Model file for the job. Use its own axes, mm. A direction names the side the tool comes from. Round coordinates to 2 decimals unless told otherwise and drop trailing zeros. Loops run counter-clockwise (first coordinate to the right, second up) from the corner with the lowest first, then second, coordinate; pieces in that order, holes last. Notation, with made-up numbers: M 22,71 L 58,71 A23 ccw 58,81 Z; hole C 88,49.25 d10. An arc over 180 degrees is marked long. Answer in a Markdown table with one row per item.
Autodesk Inventor part; units mm, degrees
ref_plane "YZ Plane" through (0, 0, 0) normal (1, 0, 0) x (0, 1, 0)
ref_plane "XZ Plane" through (0, 0, 0) normal (0, 1, 0) x (-1, 0, 0)
ref_plane "XY Plane" through (0, 0, 0) normal (0, 0, 1) x (1, 0, 0)
sketch "Эскиз1" plane through (0, 0, 0) normal (0, 1, 0) x (-1, 0, 0)
  line L0 (15, -5) -> (-15, -5)
  line L1 (-15, -5) -> (-15, 5)
  line L2 (-15, 5) -> (15, 5)
  line L3 (15, 5) -> (15, -5)
  line L4 (-15, -5) -> (15, 5) construction
  line L5 (15, -5) -> (-15, 5) construction
  line L6 (-13, -3) -> (13, -3)
  line L7 (13, -3) -> (13, 3)
  line L8 (13, 3) -> (-13, 3)
  line L9 (-13, 3) -> (-13, -3)
  point P0 (0, 0)
  point P1 (0, 0)
  dimension "d0" = 30
  dimension "d1" = 10
  dimension "d2" = 2
extrude "Выдавливание1" add sketch "Эскиз1" along normal blind 68.7
sketch "Эскиз2" plane through (15, 0, 5) normal (1, 0, 0) x (0, 0, -1)
  line L0 (0, 68.7) -> (10, 68.7) construction
  line L1 (10, 68.7) -> (0, 58.7) construction
  line L2 (0, 0) -> (0, 68.7) construction
  line L3 (0, 68.7) -> (10, 58.7) construction
  line L4 (10, 0) -> (10, 68.7) construction
  line L5 (10, 0) -> (0, 10) construction
  line L6 (0, 0) -> (10, 10) construction
  circle A0 centre (5, 63.7) radius 0.5
  circle A1 centre (5, 5) radius 0.5
  point P0 (5, 0)
  dimension "d5" = 1
  dimension "d6" = 1
sketch "Эскиз3" plane through (15, 0, -5) normal (0, 0, -1) x (-1, 0, 0)
  line L0 (0, 0) -> (0, 68.7)
  line L1 (30, 0) -> (30, 68.7)
  line L2 (30, 0) -> (30, 68.7)
  line L3 (0, 0) -> (0, 68.7)
  line L4 (0, 68.7) -> (30, 68.7)
  arc A0 (2, 58.7) -> (28, 58.7) centre (15, 58.7) ccw
  line L5 (28, 0) -> (28, 68.7)
  line L6 (2, 0) -> (2, 68.7)
  line L7 (28, 0) -> (28, 68.7)
  line L8 (28, 58.7) -> (28, 68.7)
  line L9 (28, 68.7) -> (2, 68.7)
  line L10 (2, 58.7) -> (2, 68.7)
  point P0 (15, 0)
  dimension "d10" = 10
extrude "Выдавливание3" cut sketch "Эскиз3" against normal up to surface (2 mm away)
hole "Отверстие1" at (15, 63.7, 0) at (15, 5, 0) direction (-1, 0, 0) diameter 1 depth 15 countersink diameter 1.5 countersink angle 90
mirror "Зеркальное отражение1" about plane through (0, 0, 0) normal (1, 0, 0) of "Отверстие1"
properties part number "board-1-new"
1. Tool access for faces 1 (the flat face through (0, 34, 3)), 2 (the flat face through (0, 34, 5)), 3 (the cylindrical face through (0.286, 45.703, -4.014)): list every direction of +Z, -Z, +X, -X, +Y, -Y with a clear straight run to the whole face (end or side of a thin tool).
Verdict:
| item | result |
|---|---|
| face 1 | +Y, -Y |
| face 2 | +Z, +X, -X, +Y, -Y |
| face 3 | -Z, +Y |
2. Saw through at A-A (z = 2). Write the cut outline in (x, y).
Verdict:
| item | result |
|---|---|
| outline | M -15,0 L -13,0 L -13,68.7 L -15,68.7 Z; M 13,0 L 15,0 L 15,68.7 L 13,68.7 Z |
3. Wall check: probe 1 along Y at (x, z) = (14.2, 0); probe 2 along X at (y, z) = (10, -2); probe 3 along Z at (x, y) = (-11.5, 26). Give the ranges that are in metal, low to high.
Verdict:
| item | result |
|---|---|
| probe 1 | y = 0 to 4.5, 5.5 to 63.2, 64.2 to 68.7 |
| probe 2 | x = -15 to -13, 13 to 15 |
| probe 3 | z = -5 to -3, 3 to 5 |
4. Saw through at C-C (y = 50.5). Write the cut outline in (x, z).
Verdict:
| item | result |
|---|---|
| outline | M -15,-5 L -10.09,-5 L -10.09,-3 L -13,-3 L -13,3 L 13,3 L 13,-3 L 10.09,-3 L 10.09,-5 L 15,-5 L 15,5 L -15,5 Z |
5. Saw through at B-B (x = -4.5). Write the cut outline in (y, z), and give its area (3 significant figures).
Verdict:
| item | result |
|---|---|
| outline | M 0,-5 L 46.5,-5 L 46.5,-3 L 0,-3 Z; M 0,3 L 68.7,3 L 68.7,5 L 0,5 Z |
| area | 230 mm² |
